Read the model definition and answer for the solid it produces. Units are mm, in the model's axes. Coordinates: 2 decimals unless noted, no trailing zeros. Loops run counter-clockwise (first coordinate to the right, second up) from the corner with the lowest first, then second, coordinate; pieces in that order, holes last. Notation, with made-up numbers: (27, 17.5) -> (60, 17.5) arc R38 cw to (60, 55.5) -> close; hole circle Ø6 at (56, 2.5). An arc over 180 degrees is marked (long way). Answer as CSV lines item,"result".
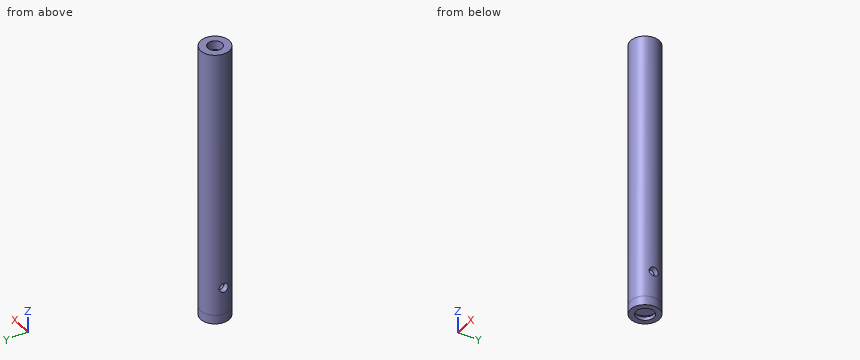
```python
from build123d import *

# Parameters (mm, degrees)
SKETCH1_R               = 8
BOSS_EXTRUDE1_DEPTH     = 150
SKETCH2_R               = 4
CUT_EXTRUDE1_DEPTH      = 5
SKETCH3_R               = 5
CUT_EXTRUDE2_DEPTH      = 135
CUT_EXTRUDE3_DEPTH      = 151.426061572
CUT_EXTRUDE3_DEPTH_BACK = 151.426061572
SKETCH4_R               = 2.5
BOSS_EXTRUDE2_START     = 5
SKETCH5_R               = 8
BOSS_EXTRUDE2_DEPTH     = 5
CUT_EXTRUDE4_START      = -2
SKETCH6_R               = 5
CUT_EXTRUDE4_DEPTH      = 2
SKETCH7_R               = 7
CUT_EXTRUDE5_DEPTH      = 2


with BuildPart() as part:
    # Sketch1 → Boss-Extrude1 (new body)
    with BuildSketch(Plane.XY):
        Circle(SKETCH1_R)
    extrude(amount=BOSS_EXTRUDE1_DEPTH)

    # Sketch2 → Cut-Extrude1 (cut)
    with BuildSketch(Plane.XY.offset(150)):
        Circle(SKETCH2_R)
    extrude(amount=-CUT_EXTRUDE1_DEPTH, mode=Mode.SUBTRACT)

    # Sketch3 → Cut-Extrude2 (cut)
    with BuildSketch(Plane.XY.offset(145)):
        Circle(SKETCH3_R)
    extrude(amount=-CUT_EXTRUDE2_DEPTH, mode=Mode.SUBTRACT)

    # Sketch4 → Cut-Extrude3 (cut, two sides: drawn at the far end of the back side and taken through both)
    with BuildSketch(Plane(origin=(0, 0, 0), x_dir=(0, 0, -1), z_dir=(1, 0, 0)).offset(-CUT_EXTRUDE3_DEPTH_BACK)):
        with Locations((-15, 0)):
            Circle(SKETCH4_R)
    extrude(amount=CUT_EXTRUDE3_DEPTH + CUT_EXTRUDE3_DEPTH_BACK, mode=Mode.SUBTRACT)

    # Sketch5 → Boss-Extrude2 (add)
    with BuildSketch(Plane(origin=(0, 0, 0), x_dir=(-1, 0, 0), z_dir=(0, 0, -1)).offset(BOSS_EXTRUDE2_START)):
        Circle(SKETCH5_R)
    extrude(amount=-BOSS_EXTRUDE2_DEPTH)

    # Sketch6 → Cut-Extrude4 (cut)
    with BuildSketch(Plane(origin=(0, 0, -5), x_dir=(-1, 0, 0), z_dir=(0, 0, -1)).offset(CUT_EXTRUDE4_START)):
        with Locations(Location((0, 0, 0), (0, 0, 180))):
            Circle(SKETCH6_R)
    extrude(amount=CUT_EXTRUDE4_DEPTH, mode=Mode.SUBTRACT)

    # Sketch7 → Cut-Extrude5 (cut)
    with BuildSketch(Plane(origin=(0, 0, -3), x_dir=(-1, 0, 0), z_dir=(0, 0, -1))):
        Circle(SKETCH7_R)
    extrude(amount=-CUT_EXTRUDE5_DEPTH, mode=Mode.SUBTRACT)


solid = part.part
```
Q1. Find the intervals of material crossed by probe 1 along Y at (x, z) = (0, -4.3); probe 2 along Z at (x, y) = (2.5, 5.5); probe 3 along Z at (x, y) = (-3, 0), in increasing order. Write a range as [from, to].
Results:
probe 1,"y = [-8, -5], [5, 8]"
probe 2,"z = [-5, -3], [-1, 150]"
probe 3,"z = [-1, 10]"
Q2. A cutting plane is placed at C-C, the plane z = 109.5. Write down the section's boundary in (x, y).
Results:
outline,"circle Ø16 at (0, 0); hole circle Ø10 at (0, 0)"
Q3. A cutting plane is placed at D-D, the plane z = 15. Write down the section's boundary in (x, y).
Results:
outline,"(-7.6, -2.5) arc R8 ccw to (7.6, -2.5) -> (4.33, -2.5) arc R5 cw to (-4.33, -2.5) -> close; (-7.6, 2.5) -> (-4.33, 2.5) arc R5 cw to (4.33, 2.5) -> (7.6, 2.5) arc R8 ccw to start"
Q4. A cutting plane is placed at A-A, the plane y = 0. Write down the section's boundary in (x, z).
Results:
outline,"(-8, -5) -> (-5, -5) -> (-5, -3) -> (-7, -3) -> (-7, -1) -> (7, -1) -> (7, -3) -> (5, -3) -> (5, -5) -> (8, -5) -> (8, 12.5) -> (5, 12.5) -> (5, 10) -> (-5, 10) -> (-5, 12.5) -> (-8, 12.5) -> close; (-8, 17.5) -> (-5, 17.5) -> (-5, 145) -> (-4, 145) -> (-4, 150) -> (-8, 150) -> close; (4, 145) -> (5, 145) -> (5, 17.5) -> (8, 17.5) -> (8, 150) -> (4, 150) -> close"
Q5. Given pin 1 Ø4 at (x, z) = (6, 52) entering from -Y; pin 2 Ø1.5 at (y, z) = (-3.5, 48) entering from +X; pin 3 Ø9 at (x, y) = (0, 0) entering from -Z, each flat-ended and moving along its own axis, determine where each tip first touches the part or whether it passes through.
Results:
pin 1,"stops at y = -6.93"
pin 2,"stops at x = 7.51"
pin 3,"stops at z = -1"
Q6. A cutting plane is placed at B-B, the plane x = 0. Write down the section's boundary in (y, z), and give its area (3 significant figures).
Results:
outline,"(-8, -5) -> (-5, -5) -> (-5, -3) -> (-7, -3) -> (-7, -1) -> (7, -1) -> (7, -3) -> (5, -3) -> (5, -5) -> (8, -5) -> (8, 150) -> (4, 150) -> (4, 145) -> (5, 145) -> (5, 10) -> (-5, 10) -> (-5, 145) -> (-4, 145) -> (-4, 150) -> (-8, 150) -> close"
area,"1,040 mm²"
